from build123d import *

# Parameters (mm, degrees)
CYLINDER013_R               = 2
CYLINDER013_DEPTH           = 12
CYLINDER013_ROLL_ANGLE      = 90
CYLINDER013_PITCH_ANGLE     = 45
CYLINDER013_PLACEMENT_ANGLE = 45
CYLINDER005_R               = 4.05
CYLINDER005_DEPTH           = 10
CYLINDER011_R               = 2
CYLINDER011_DEPTH           = 10
CYLINDER012_R               = 1.05
CYLINDER012_DEPTH           = 10
CYLINDER009_R               = 2
CYLINDER009_DEPTH           = 10
CYLINDER010_R               = 1.05
CYLINDER010_DEPTH           = 10
CYLINDER007_R               = 2
CYLINDER007_DEPTH           = 10
CYLINDER008_R               = 1.05
CYLINDER008_DEPTH           = 10
CYLINDER006_R               = 2
CYLINDER006_DEPTH           = 10
CYLINDER001_R               = 1.05
CYLINDER001_DEPTH           = 10
CYLINDER_R                  = 11
CYLINDER_DEPTH              = 9


with BuildPart() as cylinder013:
    # Cylinder013 → Cylinder013 (new body)
    with BuildSketch(Plane.XY):
        Circle(CYLINDER013_R)
    extrude(amount=CYLINDER013_DEPTH)


with BuildPart() as cylinder013_1:
    # Cylinder013 roll: moved
    add(cylinder013.part.rotate(Axis((0, 0, 0), (1, 0, 0)), CYLINDER013_ROLL_ANGLE))


with BuildPart() as cylinder013_2:
    # Cylinder013 pitch: moved
    add(cylinder013_1.part.rotate(Axis((0, 0, 0), (0, 1, 0)), CYLINDER013_PITCH_ANGLE))


with BuildPart() as cylinder013_3:
    # Cylinder013 placement: moved
    add(cylinder013_2.part.moved(Location((0, 0, 4.5))).rotate(Axis((0, 0, 4.5), (0, 0, 1)), CYLINDER013_PLACEMENT_ANGLE))


with BuildPart() as cylinder005:
    # Cylinder005 → Cylinder005 (new body)
    with BuildSketch(Plane.XY):
        Circle(CYLINDER005_R)
    extrude(amount=CYLINDER005_DEPTH)


with BuildPart() as cylinder011:
    # Cylinder011 → Cylinder011 (new body)
    with BuildSketch(Plane(origin=(8, 0, 5), x_dir=(1, 0, 0), z_dir=(0, 0, 1))):
        Circle(CYLINDER011_R)
    extrude(amount=CYLINDER011_DEPTH)


with BuildPart() as fusion003:
    # Cylinder012 → Cylinder012 (new body)
    with BuildSketch(Plane(origin=(8, 0, 0), x_dir=(1, 0, 0), z_dir=(0, 0, 1))):
        Circle(CYLINDER012_R)
    extrude(amount=CYLINDER012_DEPTH)

    # Fusion003: union Cylinder011
    add(cylinder011.part)


with BuildPart() as fusion003_1:
    # Fusion003 placement: moved
    add(fusion003.part.moved(Location((-8, -8, -1))))


with BuildPart() as cylinder009:
    # Cylinder009 → Cylinder009 (new body)
    with BuildSketch(Plane(origin=(8, 0, 5), x_dir=(1, 0, 0), z_dir=(0, 0, 1))):
        Circle(CYLINDER009_R)
    extrude(amount=CYLINDER009_DEPTH)


with BuildPart() as fusion002:
    # Cylinder010 → Cylinder010 (new body)
    with BuildSketch(Plane(origin=(8, 0, 0), x_dir=(1, 0, 0), z_dir=(0, 0, 1))):
        Circle(CYLINDER010_R)
    extrude(amount=CYLINDER010_DEPTH)

    # Fusion002: union Cylinder009
    add(cylinder009.part)


with BuildPart() as fusion002_1:
    # Fusion002 placement: moved
    add(fusion002.part.moved(Location((-8, 8, -1))))


with BuildPart() as cylinder007:
    # Cylinder007 → Cylinder007 (new body)
    with BuildSketch(Plane(origin=(8, 0, 5), x_dir=(1, 0, 0), z_dir=(0, 0, 1))):
        Circle(CYLINDER007_R)
    extrude(amount=CYLINDER007_DEPTH)


with BuildPart() as fusion001:
    # Cylinder008 → Cylinder008 (new body)
    with BuildSketch(Plane(origin=(8, 0, 0), x_dir=(1, 0, 0), z_dir=(0, 0, 1))):
        Circle(CYLINDER008_R)
    extrude(amount=CYLINDER008_DEPTH)

    # Fusion001: union Cylinder007
    add(cylinder007.part)


with BuildPart() as fusion001_1:
    # Fusion001 placement: moved
    add(fusion001.part.moved(Location((-16, 0, -1))))


with BuildPart() as cylinder006:
    # Cylinder006 → Cylinder006 (new body)
    with BuildSketch(Plane(origin=(8, 0, 5), x_dir=(1, 0, 0), z_dir=(0, 0, 1))):
        Circle(CYLINDER006_R)
    extrude(amount=CYLINDER006_DEPTH)


with BuildPart() as fusion:
    # Cylinder001 → Cylinder001 (new body)
    with BuildSketch(Plane(origin=(8, 0, 0), x_dir=(1, 0, 0), z_dir=(0, 0, 1))):
        Circle(CYLINDER001_R)
    extrude(amount=CYLINDER001_DEPTH)

    # Fusion: union Cylinder006
    add(cylinder006.part)


with BuildPart() as fusion_1:
    # Fusion placement: moved
    add(fusion.part.moved(Location((0, 0, -1))))


with BuildPart() as cut005:
    # Cylinder → Cylinder (new body)
    with BuildSketch(Plane.XY):
        Circle(CYLINDER_R)
    extrude(amount=CYLINDER_DEPTH)

    # Cut: cut Fusion
    add(fusion_1.part, mode=Mode.SUBTRACT)

    # Cut001: cut Fusion001
    add(fusion001_1.part, mode=Mode.SUBTRACT)

    # Cut002: cut Fusion002
    add(fusion002_1.part, mode=Mode.SUBTRACT)

    # Cut003: cut Fusion003
    add(fusion003_1.part, mode=Mode.SUBTRACT)

    # Cut004: cut Cylinder005
    add(cylinder005.part, mode=Mode.SUBTRACT)

    # Cut005: cut Cylinder013
    add(cylinder013_3.part, mode=Mode.SUBTRACT)


solid = cut005.part
Design review of the part built by this model. Coordinates are the model's own, in mm. A direction names the side the tool comes from. Give positions to 0.01 mm unless a question says otherwise; leave off trailing zeros. Loops run counter-clockwise (first coordinate to the right, second up) from the corner with the lowest first, then second, coordinate; pieces in that order, holes last. Notation, with made-up numbers: (10.25, 19) - (19.25, 19) arc R8 cw to (19.25, 28) - close; hole circle Ø4 at (75.5, 14). An arc over 180 degrees is marked (long way). Write item = value, one per line.
1) Take a section at C-C on z = 1.75. State the section outline as (x, y) points.
Result sheet:
outline = circle Ø22 at (0, 0); hole circle Ø2.1 at (-8, 0); hole circle Ø8.1 at (0, 0); hole circle Ø2.1 at (0, -8); hole circle Ø2.1 at (0, 8); hole circle Ø2.1 at (8, 0)
2) Clearance check with flat-ended pins moving along their axes: pin 1 Ø5 at (x, y) = (0, 0) entering from -Z; pin 2 Ø1 at (x, z) = (4.5, 3.5) entering from +Y; pin 3 Ø2 at (y, z) = (-7, 5.5) entering from -X; pin 4 Ø4 at (y, z) = (-3, 6.5) entering from -X. State where each tip first meets the part, or that it passes through.
Result sheet:
pin_1 = through
pin_2 = 10.25
pin_3 = -9.22
pin_4 = -10.95
3) Take a section at A-A on y = 0. State the section outline as (x, z) points.
Result sheet:
outline = (-11, 0) - (-9.05, 0) - (-9.05, 4) - (-10, 4) - (-10, 9) - (-11, 9) - close; (-6.95, 0) - (-4.05, 0) - (-4.05, 9) - (-6, 9) - (-6, 4) - (-6.95, 4) - close; (4.05, 0) - (6.95, 0) - (6.95, 4) - (6, 4) - (6, 9) - (4.05, 9) - close; (9.05, 0) - (11, 0) - (11, 9) - (10, 9) - (10, 4) - (9.05, 4) - close
4) To check wall thickness, follow line 1 (Y direction, x = 0, z = 5.6); line 2 (Y direction, x = 0, z = 1.55); line 3 (X direction, y = -0.75, z = 7.75). State the ranges of each line that lie inside material, in increasing order.
Result sheet:
line_1 = -11 to -10, -6 to -4.05, 4.05 to 6, 10 to 11
line_2 = -11 to -9.05, -6.95 to -4.05, 4.05 to 6.95, 9.05 to 11
line_3 = -10.97 to -9.85, -6.15 to -3.98, 3.98 to 6.15, 9.85 to 10.97
5) Tool access review of faces 4 (the face through (1, -9, 4)), 5 (the face through (-2.985, 2.737, 4.437)): name each direction out of +Z, -Z, +X, -X, +Y, -Y from which nothing blocks a thin tool from reaching the whole face with its end or side.
Result sheet:
face_4 = +Z
face_5 = +Z, -Z
6) Take a section at D-D on x = -3.75. State the section outline as (y, z) points.
Result sheet:
outline = (-10.34, 0) - (-1.53, 0) - (-1.53, 9) - (-10.34, 9) - close; (1.53, 0) - (10.34, 0) - (10.34, 9) - (1.53, 9) - close
7) Draft analysis for pull direction X (two halves, no side actions). For faces 1 (the face through (0.56, 8.89, 1.97)), 2 (the face through (-2.38, -10.74, 4.44)), 3 (the face through (0, -5, 9)), state which applies: +X half, -X half, draft (parallel to the pull), parting line (faces both ways), or undercut.
Result sheet:
face_1 = undercut
face_2 = parting line
face_3 = draft
